from build123d import *

# Parameters (mm, degrees)
F1_DEPTH = 2298.7


with BuildPart() as f1:
    # F0 (on Top) → F1 (new body)
    with BuildSketch(Plane.XY):
        with BuildLine():
            Line((-50.8, 0), (50.8, 0))
            Line((50.8, 0), (50.8, 6.35))
            ThreePointArc((50.8, 6.35), (64.270384, 11.929616), (69.85, 25.4))
            Line((69.85, 25.4), (76.2, 25.4))
            Line((76.2, 25.4), (76.2, 127))
            Line((76.2, 127), (69.85, 127))
            ThreePointArc((69.85, 127), (64.270384, 140.470384), (50.8, 146.05))
            Line((50.8, 146.05), (50.8, 152.4))
            Line((50.8, 152.4), (-50.8, 152.4))
            Line((-50.8, 152.4), (-50.8, 146.05))
            ThreePointArc((-50.8, 146.05), (-64.270384, 140.470384), (-69.85, 127))
            Line((-69.85, 127), (-76.2, 127))
            Line((-76.2, 127), (-76.2, 25.4))
            Line((-76.2, 25.4), (-69.85, 25.4))
            ThreePointArc((-69.85, 25.4), (-64.270384, 11.929616), (-50.8, 6.35))
            Line((-50.8, 6.35), (-50.8, 0))
        make_face()
    extrude(amount=F1_DEPTH)


solid = f1.part
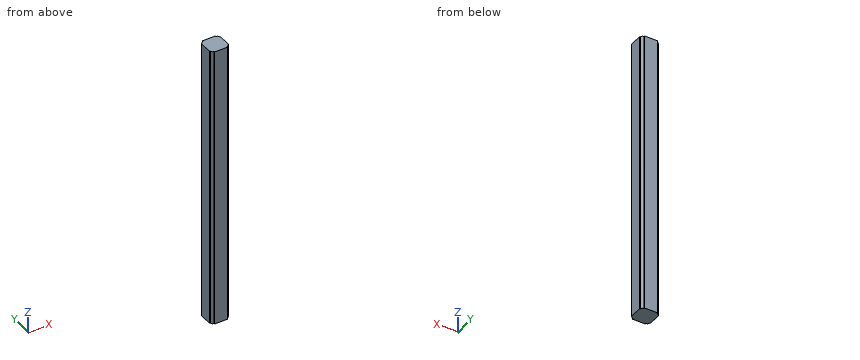
Geometry check sheet. Reference: the model listing, model coordinates, mm. Give positions to 0.01 mm unless a question says otherwise; leave off trailing zeros. Loops run counter-clockwise (first coordinate to the right, second up) from the corner with the lowest first, then second, coordinate; pieces in that order, holes last. Notation, with made-up numbers: M 39,-38.75 L 82,-38.75 A19 ccw 82,-30.75 Z; hole C 14,83.25 d6. An arc over 180 degrees is marked long. Write each question's results on one line, items separated by ' | '.
1) Thickness scan on line 1 (X direction, y = 130, z = 1988.5); line 2 (Y direction, x = -51, z = 1446); line 3 (X direction, y = 135, z = 1496). Record the ranges inside material, lowest first.
Answers follow:
line 1: -69.61 to 69.61 | line 2: 6.35 to 146.05 | line 3: -68.09 to 68.09
2) Section check A-A, the plane z = 403. Record the boundary of the cut face in (x, y).
Answers follow:
outline: M -76.2,25.4 L -69.85,25.4 A19.05 ccw -50.8,6.35 L -50.8,0 L 50.8,0 L 50.8,6.35 A19.05 ccw 69.85,25.4 L 76.2,25.4 L 76.2,127 L 69.85,127 A19.05 ccw 50.8,146.05 L 50.8,152.4 L -50.8,152.4 L -50.8,146.05 A19.05 ccw -69.85,127 L -76.2,127 Z
3) Gauge pin test, flat ends, axial feed: pin 1 (3 mm diameter, centred on y = 150.5, z = 1654, fed in from -X); pin 2 (7 mm diameter, centred on x = 73.5, z = 1223.5, fed in from +Y); pin 3 (1.9 mm diameter, centred on x = -74, z = 963, fed in from -Y). Record the tip position at first contact, or that the pin passes through.
Answers follow:
pin 1: x = -50.8 | pin 2: y = 127 | pin 3: y = 25.4
